```python
from build123d import *

# Parameters (mm, degrees)
SKETCH_1_R          = 9.5
EXTRUDE_1_DEPTH     = 25
SKETCH_2_R          = 4
CUT_EXTRUDE_1_DEPTH = 12.5
SKETCH_3_R          = 3
CUT_EXTRUDE_2_DEPTH = 12.5


with BuildPart() as part:
    # 草图1 → 凸台-拉伸1 (new body)
    with BuildSketch(Plane.XY):
        Circle(SKETCH_1_R)
    extrude(amount=EXTRUDE_1_DEPTH)

    # 草图2 → 切除-拉伸1 (cut)
    with BuildSketch(Plane.XY.offset(25)):
        Circle(SKETCH_2_R)
    extrude(amount=-CUT_EXTRUDE_1_DEPTH, mode=Mode.SUBTRACT)

    # 草图3 → 切除-拉伸2 (cut)
    with BuildSketch(Plane(origin=(0, 0, 0), x_dir=(-1, 0, 0), z_dir=(0, 0, -1))):
        Circle(SKETCH_3_R)
    extrude(amount=-CUT_EXTRUDE_2_DEPTH, mode=Mode.SUBTRACT)


solid = part.part
```
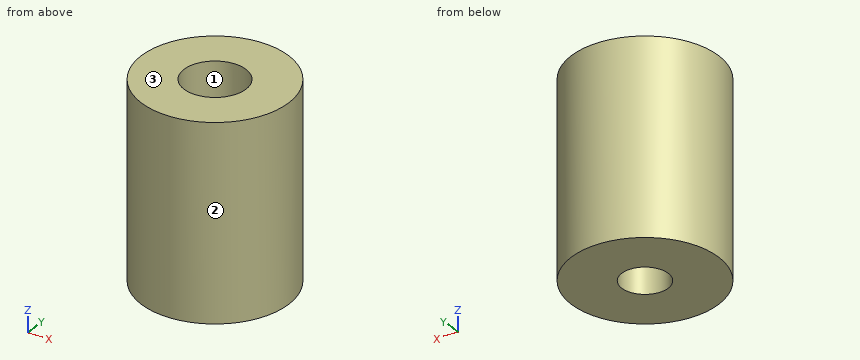
Model file for the job. Use its own axes, mm. Face numbers are marked on the shaded views. Coordinates: 2 decimals unless noted, no trailing zeros. Order: outer loops, then holes, each group sorted by start corner. A loop starts at its lowest first (then second) coordinate and runs counter-clockwise, first axis right, second up. Notation, with made-up numbers: (41, -12) -> (78, -12) arc R16 cw to (78, 2) -> close; hole circle Ø2 at (11.25, 52.5). An arc over 180 degrees is marked (long way). Return JSON: item names as keys, results as strings.
Item 1: Wall check: line 1 along Y through (x, z) = (0, 20.25); line 2 along Y through (x, z) = (0, 8.5); line 3 along X through (y, z) = (-1.75, 3.5). Give the ranges that are in metal, low to high. Write a range as from..to.
Model answer:
{"line 1": "y = -9.5..-4, 4..9.5", "line 2": "y = -9.5..-3, 3..9.5", "line 3": "x = -9.34..-2.44, 2.44..9.34"}
Item 2: Slice it at A-A (x = 0). Write the cut outline in (y, z).
Model answer:
{"outline": "(-9.5, 0) -> (-3, 0) -> (-3, 12.5) -> (-4, 12.5) -> (-4, 25) -> (-9.5, 25) -> close; (3, 0) -> (9.5, 0) -> (9.5, 25) -> (4, 25) -> (4, 12.5) -> (3, 12.5) -> close"}
Item 3: Slice it at C-C (z = 21). Write the cut outline in (x, y), then the cut area to 3 significant figures.
Model answer:
{"outline": "circle Ø19 at (0, 0); hole circle Ø8 at (0, 0)", "area": "233 mm²"}
Item 4: Pin check, flat tips, straight feed: P1, Ø6, axis at x = 3.5, z = 13, coming from the +Y side; P2, Ø5, axis at y = -1, z = 13, coming from the -X side; P3, Ø10, axis at x = -7, z = 21.5, coming from the +Y side; P4, Ø2, axis at y = 5, z = 22, coming from the -X side. Stop position of each tip, or through.
Model answer:
{"P1": "stops at y = 9.49", "P2": "stops at x = -9.5", "P3": "stops at y = 9.29", "P4": "stops at x = -8.62"}
Item 5: Mould opens along Y. For the marked faces 1, 2 and 3 say: pulls with the +Y half, pulls with the -Y half, needs draft (parallel to the pull), parting line crosses it, or undercut.
Model answer:
{"face 1": "undercut", "face 2": "parting line crosses it", "face 3": "needs draft"}
Item 6: Slice it at D-D (y = 4.5). Write the cut outline in (x, z).
Model answer:
{"outline": "(-8.37, 0) -> (8.37, 0) -> (8.37, 25) -> (-8.37, 25) -> close"}
